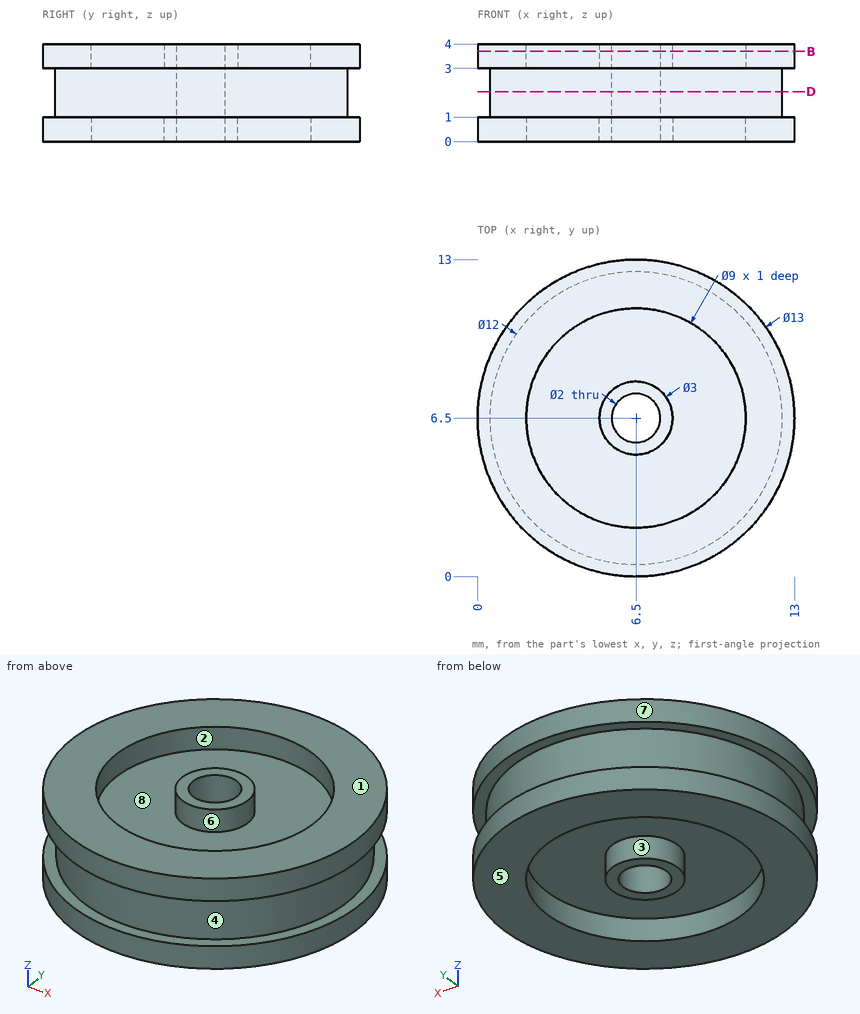
Geometry check sheet. Reference: drawing and pictorial views, mm from the part's lowest x, y, z. A direction names the side the tool comes from. Give positions to 0.01 mm unless a question says otherwise; leave off trailing zeros. Order: outer loops, then holes, each group sorted by start corner. A loop starts at its lowest first (then second) coordinate and runs counter-clockwise, first axis right, second up. Notation, with made-up numbers: (25, 68.5) - (84, 68.5) arc R13 ccw to (84, 72.5) - close; hole circle Ø2 at (7.5, -39.5). An arc over 180 degrees is marked (long way). Use one line per item in the form item = value.
1) Depth check by flat-ended pin: pin 1 Ø5.5 at (x, y) = (6.5, 6.5) entering from -Z; pin 2 Ø1.5 at (x, y) = (4.5, 5) entering from +Z. Enter the tip coordinate at first touch or a pass-through.
Working result:
pin_1 = 0
pin_2 = 3
2) Sectioned sample at D-D (z = 2.05). Record the boundary of the cut face in (x, y).
Working result:
outline = circle Ø12 at (6.5, 6.5); hole circle Ø2 at (6.5, 6.5)
3) Access from +Z, -Z, +X, -X, +Y, -Y to the whole of each face (thin tool, end or side, straight path). Record for the marked faces 1, 2, 3 and 4.
Working result:
face_1 = +Z, +X, -X, +Y, -Y
face_2 = +Z
face_3 = -Z
face_4 = none
4) Sectioned sample at B-B (z = 3.7). Record the boundary of the cut face in (x, y).
Working result:
outline = circle Ø13 at (6.5, 6.5); circle Ø3 at (6.5, 6.5); hole circle Ø9 at (6.5, 6.5); hole circle Ø2 at (6.5, 6.5)
5) Material ranges on probe 1 along Y at (x, z) = (6.5, 0.3); probe 2 along Z at (x, y) = (11.25, 2.25); probe 3 along Z at (x, y) = (9, 3.5), recorded low to high. Write a range as from..to.
Working result:
probe_1 = 0..2, 5..5.5, 7.5..8, 11..13
probe_2 = 0..1, 3..4
probe_3 = 1..3
6) Draft check along X on the marked faces 5, 6, 7 and 8. Enter one of: released by +X, released by -X, zero draft, split by the parting line, or undercut.
Working result:
face_5 = zero draft
face_6 = undercut
face_7 = split by the parting line
face_8 = undercut
